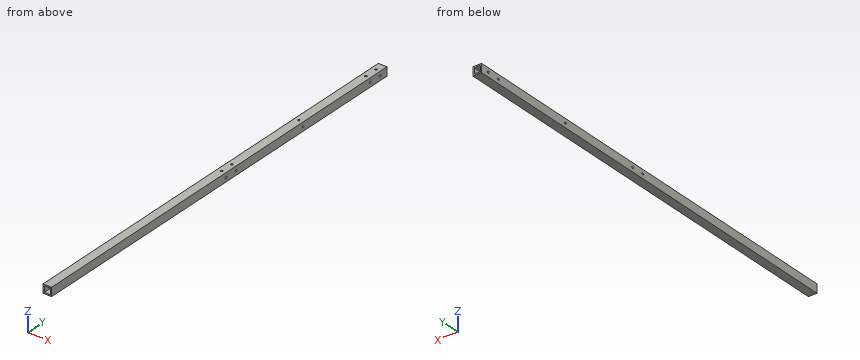
from build123d import *

# Parameters (mm, degrees)
SKETCH1_W                   = 20
SKETCH1_H                   = 20
SKETCH1_W_2                 = 14
SKETCH1_H_2                 = 14
BOSS_EXTRUDE1_DEPTH         = 1000
SKETCH3_R                   = 2.5
CUT_EXTRUDE1_DEPTH          = 10
LPATTERN1_COUNT             = 3
LPATTERN1_PITCH             = 230
CIRPATTERN1_COUNT           = 3
CIRPATTERN1_ANGLE           = 180
CIRPATTERN1_COPY_1_SKETCH_R = 2.5
CIRPATTERN1_COPY_1_DEPTH    = 10
CIRPATTERN1_COPY_2_SKETCH_R = 2.5
CIRPATTERN1_COPY_2_DEPTH    = 10
CIRPATTERN1_COPY_3_SKETCH_R = 2.5
CIRPATTERN1_COPY_3_DEPTH    = 10
CIRPATTERN1_COPY_4_SKETCH_R = 2.5
CIRPATTERN1_COPY_4_DEPTH    = 10
SKETCH6_R                   = 2.5
CUT_EXTRUDE2_DEPTH          = 10
LPATTERN2_COUNT             = 2
LPATTERN2_PITCH             = 400
CIRPATTERN2_COUNT           = 3
CIRPATTERN2_ANGLE           = 180
CIRPATTERN2_COPY_1_SKETCH_R = 2.5
CIRPATTERN2_COPY_1_DEPTH    = 10
CIRPATTERN2_COPY_2_SKETCH_R = 2.5
CIRPATTERN2_COPY_2_DEPTH    = 10


with BuildPart() as part:
    # Sketch1 → Boss-Extrude1 (new body)
    with BuildSketch(Plane(origin=(0, 0, 0), x_dir=(1, 0, 0), z_dir=(0, 1, 0))):
        with Locations((10, 10)):
            Rectangle(SKETCH1_W, SKETCH1_H)
        with Locations((10, 10)):
            Rectangle(SKETCH1_W_2, SKETCH1_H_2, mode=Mode.SUBTRACT)
    extrude(amount=BOSS_EXTRUDE1_DEPTH)

    # Sketch3 → Cut-Extrude1 (cut)
    with BuildSketch(Plane(origin=(20, 0, 0), x_dir=(0, 0, -1), z_dir=(1, 0, 0))):
        with Locations((10, 980)):
            Circle(SKETCH3_R)
    cut_extrude1 = extrude(amount=-CUT_EXTRUDE1_DEPTH, mode=Mode.SUBTRACT)

    # LPattern1: Cut-Extrude1 ×3
    with Locations(*[(0, -i * LPATTERN1_PITCH, 0) for i in range(1, LPATTERN1_COUNT)]):
        add(cut_extrude1, mode=Mode.SUBTRACT)

    # CirPattern1: Cut-Extrude1 ×3 about axis
    cirpattern1_axis = Axis((10, 1000, -10), (0, -1, 0))
    for i in range(1, CIRPATTERN1_COUNT):
        add(cut_extrude1.rotate(cirpattern1_axis, i * CIRPATTERN1_ANGLE / (CIRPATTERN1_COUNT - 1)), mode=Mode.SUBTRACT)

    # CirPattern1 copy 1 sketch → CirPattern1 copy 1 (cut)
    with BuildSketch(Plane(origin=(0, -230, 0), x_dir=(1, 0, 0), z_dir=(0, 0, 1))):
        with Locations((10, 980)):
            Circle(CIRPATTERN1_COPY_1_SKETCH_R)
    extrude(amount=-CIRPATTERN1_COPY_1_DEPTH, mode=Mode.SUBTRACT)

    # CirPattern1 copy 2 sketch → CirPattern1 copy 2 (cut)
    with BuildSketch(Plane(origin=(0, -230, -20), x_dir=(0, 0, 1), z_dir=(-1, 0, 0))):
        with Locations((10, 980)):
            Circle(CIRPATTERN1_COPY_2_SKETCH_R)
    extrude(amount=-CIRPATTERN1_COPY_2_DEPTH, mode=Mode.SUBTRACT)

    # CirPattern1 copy 3 sketch → CirPattern1 copy 3 (cut)
    with BuildSketch(Plane(origin=(0, -460, 0), x_dir=(1, 0, 0), z_dir=(0, 0, 1))):
        with Locations((10, 980)):
            Circle(CIRPATTERN1_COPY_3_SKETCH_R)
    extrude(amount=-CIRPATTERN1_COPY_3_DEPTH, mode=Mode.SUBTRACT)

    # CirPattern1 copy 4 sketch → CirPattern1 copy 4 (cut)
    with BuildSketch(Plane(origin=(0, -460, -20), x_dir=(0, 0, 1), z_dir=(-1, 0, 0))):
        with Locations((10, 980)):
            Circle(CIRPATTERN1_COPY_4_SKETCH_R)
    extrude(amount=-CIRPATTERN1_COPY_4_DEPTH, mode=Mode.SUBTRACT)

    # Sketch6 → Cut-Extrude2 (cut)
    with BuildSketch(Plane(origin=(20, 0, 0), x_dir=(0, 0, -1), z_dir=(1, 0, 0))):
        with Locations((10, 950)):
            Circle(SKETCH6_R)
    cut_extrude2 = extrude(amount=-CUT_EXTRUDE2_DEPTH, mode=Mode.SUBTRACT)

    # LPattern2: Cut-Extrude2 ×2
    with Locations(*[(0, -i * LPATTERN2_PITCH, 0) for i in range(1, LPATTERN2_COUNT)]):
        add(cut_extrude2, mode=Mode.SUBTRACT)

    # CirPattern2: Cut-Extrude2 ×3 about axis
    cirpattern2_axis = Axis((10, 1000, -10), (0, -1, 0))
    for i in range(1, CIRPATTERN2_COUNT):
        add(cut_extrude2.rotate(cirpattern2_axis, i * CIRPATTERN2_ANGLE / (CIRPATTERN2_COUNT - 1)), mode=Mode.SUBTRACT)

    # CirPattern2 copy 1 sketch → CirPattern2 copy 1 (cut)
    with BuildSketch(Plane(origin=(0, -400, 0), x_dir=(1, 0, 0), z_dir=(0, 0, 1))):
        with Locations((10, 950)):
            Circle(CIRPATTERN2_COPY_1_SKETCH_R)
    extrude(amount=-CIRPATTERN2_COPY_1_DEPTH, mode=Mode.SUBTRACT)

    # CirPattern2 copy 2 sketch → CirPattern2 copy 2 (cut)
    with BuildSketch(Plane(origin=(0, -400, -20), x_dir=(0, 0, 1), z_dir=(-1, 0, 0))):
        with Locations((10, 950)):
            Circle(CIRPATTERN2_COPY_2_SKETCH_R)
    extrude(amount=-CIRPATTERN2_COPY_2_DEPTH, mode=Mode.SUBTRACT)


solid = part.part
Work out the finished part from the listing and answer in its coordinate system (mm). Give positions to 0.01 mm unless a question says otherwise; leave off trailing zeros. Loops run counter-clockwise (first coordinate to the right, second up) from the corner with the lowest first, then second, coordinate; pieces in that order, holes last. Notation, with made-up numbers: (35, 37) -> (55, 37) arc R10 ccw to (55, 47) -> close; hole circle Ø5 at (26, 66). An arc over 180 degrees is marked (long way). Use a Markdown table: item, result. Add a question column.
1) Each of these flat-tipped pins is pushed along its axis until it touches: P1, Ø5, axis at x = 10.5, y = 582, coming from the +Z side; P2, Ø4.5, axis at x = 10, y = 520, coming from the +Z side. Where does it stop, or does it pass through?
2) The part is cut by section A-A, the plane y = 127. Determine the outline of the cut face in (x, z), plus the area to 3 significant figures.
3) Consider line 1 along Y through (x, z) = (10, -1.4); line 2 along Z through (x, y) = (10.5, 937); line 3 along X through (y, z) = (360.5, -10.5). Determine where each line is inside the solid, lowest interval first.
Reported:
| question | item | result |
|---|---|---|
| 1 | P1 | stops at z = 0 |
| 1 | P2 | stops at z = -17 |
| 2 | outline | (0, -20) -> (20, -20) -> (20, 0) -> (0, 0) -> close; hole (3, -17) -> (17, -17) -> (17, -3) -> (3, -3) -> close |
| 2 | area | 204 mm^2 |
| 3 | line 1 | y = 0 to 517.5, 522.5 to 547.5, 552.5 to 747.5, 752.5 to 947.5, 952.5 to 977.5, 982.5 to 1000 |
| 3 | line 2 | z = -20 to -17, -3 to 0 |
| 3 | line 3 | x = 0 to 3, 17 to 20 |
